Work out the finished part from the listing and answer in its coordinate system (mm). A direction names the side the tool comes from. Coordinates: 2 decimals unless noted, no trailing zeros. Order: outer loops, then holes, each group sorted by start corner. A loop starts at its lowest first (then second) coordinate and runs counter-clockwise, first axis right, second up. Notation, with made-up numbers: (17, -36.75) - (74, -36.75) arc R18 cw to (74, -16.75) - close; hole circle Ø8 at (7, 33). An arc over 180 degrees is marked (long way). Use CSV: the item, a comma, the result in double quotes. Start each with the question number.
from build123d import *

# Parameters (mm, degrees)
BOSS_EXTRUDE1_DEPTH = 3
SKETCH2_R           = 1
CUT_EXTRUDE1_DEPTH  = 6
SKETCH3_R           = 1.5
CUT_EXTRUDE2_DEPTH  = 10


with BuildPart() as part:
    # Sketch1 → Boss-Extrude1 (new body)
    with BuildSketch(Plane(origin=(0, 0, 0), x_dir=(1, 0, 0), z_dir=(0, 1, 0))):
        Polygon((-43.75, 22.25), (-31.25, 22.25), (-31.25, 44), (31.25, 44), (31.25, 22.25), (43.75, 22.25), (43.75, 17.75), (31.25, 17.75), (31.25, -17.75), (43.75, -17.75), (43.75, -22.25), (31.25, -22.25), (31.25, -44), (-31.25, -44), (-31.25, -22.25), (-43.75, -22.25), (-43.75, -17.75), (-31.25, -17.75), (-31.25, 17.75), (-43.75, 17.75), align=None)
    extrude(amount=BOSS_EXTRUDE1_DEPTH)

    # Sketch2 → Cut-Extrude1 (cut)
    with BuildSketch(Plane.XZ):
        with Locations((-41.25, 20)):
            Circle(SKETCH2_R)
        with Locations((-41.25, -20)):
            Circle(SKETCH2_R)
        with Locations((41.25, -20)):
            Circle(SKETCH2_R)
        with Locations((41.25, 20)):
            Circle(SKETCH2_R)
    extrude(amount=-CUT_EXTRUDE1_DEPTH, mode=Mode.SUBTRACT)

    # Sketch3 → Cut-Extrude2 (cut)
    with BuildSketch(Plane(origin=(0, 3, 0), x_dir=(1, 0, 0), z_dir=(0, 1, 0))):
        with Locations((-16, 32)):
            Circle(SKETCH3_R)
        with Locations((16, 32)):
            Circle(SKETCH3_R)
        with Locations((16, -32)):
            Circle(SKETCH3_R)
        with Locations((-16, -32)):
            Circle(SKETCH3_R)
    extrude(amount=-CUT_EXTRUDE2_DEPTH, mode=Mode.SUBTRACT)


solid = part.part
1) For faces 1 (the face through (31.25, 1, -33)), 2 (the face through (-31.25, 1, 0)), 3 (the face through (-31.25, 1, -33)), determine the directions among +Z, -Z, +X, -X, +Y, -Y from which every point of the face is accessible in a straight line to the end or side of a thin tool.
2) Flat-ended cylindrical pins translate along their axes: P1, Ø0.9, axis at y = 2, z = 33, coming from the +X side; P2, Ø1.6, axis at x = 41.25, z = -20, coming from the -Y side (3 decimals); P3, Ø1.5, axis at y = 1.5, z = -27.5, coming from the -X side; P4, Ø0.9, axis at x = 34.5, y = 2, coming from the +Z side. Find the tip coordinate at first contact, or state that the pin passes through.
3) The part is cut by section A-A on x = -16. Determine the outline of the cut face in (y, z).
4) For a pull along Z with two mould halves and no side action, classify faces 4 (the face through (0, 1, -44)), 5 (the face through (-17.5, 1.52, -32.07)), 6 (the face through (-37, 1, 22.25)), 7 (the face through (-31.25, 1, 33)) as +Z half, -Z half, draft (parallel to the pull), parting line (faces both ways), or undercut.
5) Straight lines are drawn through the part: line 1 (X direction, y = 1.7, z = -32); line 2 (Z direction, x = 16, y = 2.3); line 3 (Z direction, x = -41.25, y = 0.95). For each, find the intervals that lie inside material, in ascending order. Write a range as [from, to].
6) The part is cut by section C-C on z = 20. Determine the outline of the cut face in (x, y), plus the area to 4 significant figures.
7) The part is cut by section D-D on y = 1.4. State how many separate pieces and enclosed holes the cut face has, plus the area to 3 significant figures.
8) The part is cut by section B-B on x = 36.5. Determine the outline of the cut face in (y, z), plus the area to 3 significant figures.
Answer key:
1,face 1,"-Z, +X, +Y, -Y"
1,face 2,"-X, +Y, -Y"
1,face 3,"-Z, -X, +Y, -Y"
2,P1,"x = 31.25"
2,P2,"through"
2,P3,"x = -31.25"
2,P4,"z = 22.25"
3,outline,"(0, -44) - (3, -44) - (3, -33.5) - (0, -33.5) - close; (0, -30.5) - (3, -30.5) - (3, 30.5) - (0, 30.5) - close; (0, 33.5) - (3, 33.5) - (3, 44) - (0, 44) - close"
4,face 4,"-Z half"
4,face 5,"undercut"
4,face 6,"+Z half"
4,face 7,"draft"
5,line 1,"[-31.25, -17.5], [-14.5, 14.5], [17.5, 31.25]"
5,line 2,"[-44, -33.5], [-30.5, 30.5], [33.5, 44]"
5,line 3,"[-22.25, -21], [-19, -17.75], [17.75, 19], [21, 22.25]"
6,outline,"(-43.75, 0) - (-42.25, 0) - (-42.25, 3) - (-43.75, 3) - close; (-40.25, 0) - (40.25, 0) - (40.25, 3) - (-40.25, 3) - close; (42.25, 0) - (43.75, 0) - (43.75, 3) - (42.25, 3) - close"
6,area,"250.5 mm^2"
7,separate pieces,"1"
7,enclosed holes,"8"
7,area,"5,680 mm^2"
8,outline,"(0, -22.25) - (3, -22.25) - (3, -17.75) - (0, -17.75) - close; (0, 17.75) - (3, 17.75) - (3, 22.25) - (0, 22.25) - close"
8,area,"27.0 mm^2"
